Verification items for the finished model (mm, model axes). Face numbers are marked on the shaded views. Give positions to 0.01 mm unless a question says otherwise; leave off trailing zeros. Loops run counter-clockwise (first coordinate to the right, second up) from the corner with the lowest first, then second, coordinate; pieces in that order, holes last. Notation, with made-up numbers: M -34.5,86.25 L -18.5,86.25 A18 ccw -18.5,95.25 Z; hole C 49,37.25 d10. An arc over 180 degrees is marked long. Answer in a Markdown table with one row per item.
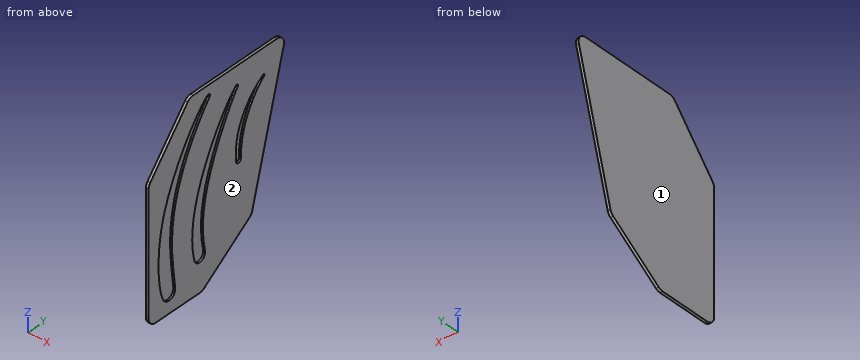
```python
from build123d import *

# Parameters (mm, degrees)
BOSS_EXTRUDE1_DEPTH = 10
CUT_EXTRUDE2_DEPTH  = 7


with BuildPart() as part:
    # Sketch1 → Boss-Extrude1 (new body)
    with BuildSketch(Plane(origin=(0, 0, 0), x_dir=(0, 0, -1), z_dir=(1, 0, 0))):
        with BuildLine():
            Line((0, -39.159060238), (0, -399.159060238))
            ThreePointArc((0, -399.159060238), (2.810766389, -411.83760809), (10.716371709, -422.140393531))
            Line((10.716371709, -422.140393531), (202.227482489, -582.837295953))
            ThreePointArc((202.227482489, -582.837295953), (211.25050648, -588.046741283), (221.51111078, -589.855962659))
            Line((221.51111078, -589.855962659), (671.51111078, -589.855962659))
            ThreePointArc((671.51111078, -589.855962659), (692.724314215, -581.069166095), (701.51111078, -559.855962659))
            Line((701.51111078, -559.855962659), (701.51111078, -369.855962659))
            ThreePointArc((701.51111078, -369.855962659), (700.081380744, -360.705024227), (695.928465834, -352.426310564))
            Line((695.928465834, -352.426310564), (556.491249073, -157.087470131))
            ThreePointArc((556.491249073, -157.087470131), (549.188422732, -149.877866821), (539.883012979, -145.551320648))
            Line((539.883012979, -145.551320648), (37.809118961, -10.19325866))
            ThreePointArc((37.809118961, -10.19325866), (11.755460664, -15.344426409), (0, -39.159060238))
        make_face()
    extrude(amount=BOSS_EXTRUDE1_DEPTH)

    # Sketch4 → Cut-Extrude2 (cut)
    with BuildSketch(Plane(origin=(10, 0, 0), x_dir=(0, 0, -1), z_dir=(1, 0, 0))):
        with BuildLine():
            ThreePointArc((646.133694128, -523.626722446), (654.270375926, -492.315038086), (626.364411935, -475.947865394))
            add(Edge.make_bspline(
                [(626.364411935, -475.947865394), (572.427382245, -482.279425386), (369.496171973, -510.067463814), (179.998241324, -434.657283692), (42.396217675, -327.560917886)],
                knots=[0, 0, 0, 0, 0.257311007, 1, 1, 1, 1], degree=3))
            ThreePointArc((42.396217675, -327.560917886), (38.301805286, -326.1553415), (34.207392898, -327.560917886))
            add(Edge.make_bspline(
                [(34.207392898, -327.560917886), (14.475713482, -342.918185901), (324.808789115, -589.015611509), (620.265200397, -544.090123727), (646.133694128, -523.626722446)],
                knots=[0, 0, 0, 0, 0.545719307, 1, 1, 1, 1], degree=3))
        make_face()
        with BuildLine():
            ThreePointArc((332.693478174, -215.359019498), (341.545058852, -204.318697463), (331.179728441, -194.685467652))
            add(Edge.make_bspline(
                [(331.179728441, -194.685467652), (300.184384568, -194.688304583), (192.730208888, -182.13783781), (112.622758483, -114.88285895), (98.829146805, -93.988930122)],
                knots=[0, 0, 0, 0, 0.339117248, 1, 1, 1, 1], degree=3))
            ThreePointArc((98.829146805, -93.988930122), (93.433821546, -92.827514339), (92.163413905, -98.198220596))
            add(Edge.make_bspline(
                [(92.163413905, -98.198220596), (126.325036043, -154.802617957), (226.918714052, -224.562098265), (331.921739283, -215.472572374), (332.693478174, -215.359019498)],
                knots=[0, 0, 0, 0, 0.645739259, 1, 1, 1, 1], degree=3))
        make_face()
        with BuildLine():
            ThreePointArc((74.202765192, -208.284508838), (67.092959072, -208.260098077), (66.698936736, -215.359019498))
            add(Edge.make_bspline(
                [(66.698936736, -215.359019498), (100.320017518, -254.957400328), (300.322217315, -390.035120939), (509.639726303, -410.500517765), (577.755509271, -393.526935767)],
                knots=[0, 0, 0, 0, 0.654710405, 1, 1, 1, 1], degree=3))
            ThreePointArc((577.755509271, -393.526935767), (594.800287265, -365.58541059), (567.085033992, -348.175125638))
            add(Edge.make_bspline(
                [(567.085033992, -348.175125638), (526.742508558, -357.109499901), (316.076431581, -369.790908175), (81.149231878, -214.924232147), (74.202765192, -208.284508838)],
                knots=[0, 0, 0, 0, 0.231564943, 1, 1, 1, 1], degree=3))
        make_face()
    extrude(amount=-CUT_EXTRUDE2_DEPTH, mode=Mode.SUBTRACT)


solid = part.part
```
Item 1: Scan lines: L1, parallel to Y at x = 3.25, z = -397; L2, parallel to Y at x = 6.25, z = -250.5; L3, parallel to Y at x = 5.25, z = -549.5. Record each from-to range of solid material in increasing order. Write a range as [from, to].
Reported:
| item | result |
|---|---|
| L1 | y = [-589.86, -536.46], [-485.68, -390.78], [-349.2, -107.03] |
| L2 | y = [-589.86, -487.37], [-448.7, -337.74], [-303.26, -210.49], [-185.42, -67.53] |
| L3 | y = [-589.86, -546.16], [-484.81, -399.18], [-351.59, -150.1] |
Item 2: Release check for a two-part mould opening along X. For the marked faces 1 and 2 record: released by +X, released by -X, zero draft, split by the parting line, or undercut.
Reported:
| item | result |
|---|---|
| face 1 | released by -X |
| face 2 | released by +X |
Item 3: Go/stop test with flat-tipped pins: pin 1 (5 mm diameter, centred on x = 5, z = -112.5, fed in from +Y); pin 2 (6 mm diameter, centred on x = 8.5, y = -220, fed in from -Z). Record where each tip stops, or that it passes through.
Reported:
| item | result |
|---|---|
| pin 1 | stops at y = -29.66 |
| pin 2 | stops at z = -603.54 |
Item 4: Sectioned sample at A-A (x = 7.5). State how many separate pieces and enclosed holes the cut face has, and give its area (3 significant figures).
Reported:
| item | result |
|---|---|
| separate pieces | 1 |
| enclosed holes | 3 |
| area | 263,000 mm^2 |
Item 5: Sectioned sample at B-B (y = -71). Record the cut outline in (x, z).
Reported:
| item | result |
|---|---|
| outline | M 0,-263.36 L 10,-263.36 L 10,0 L 0,0 Z |
